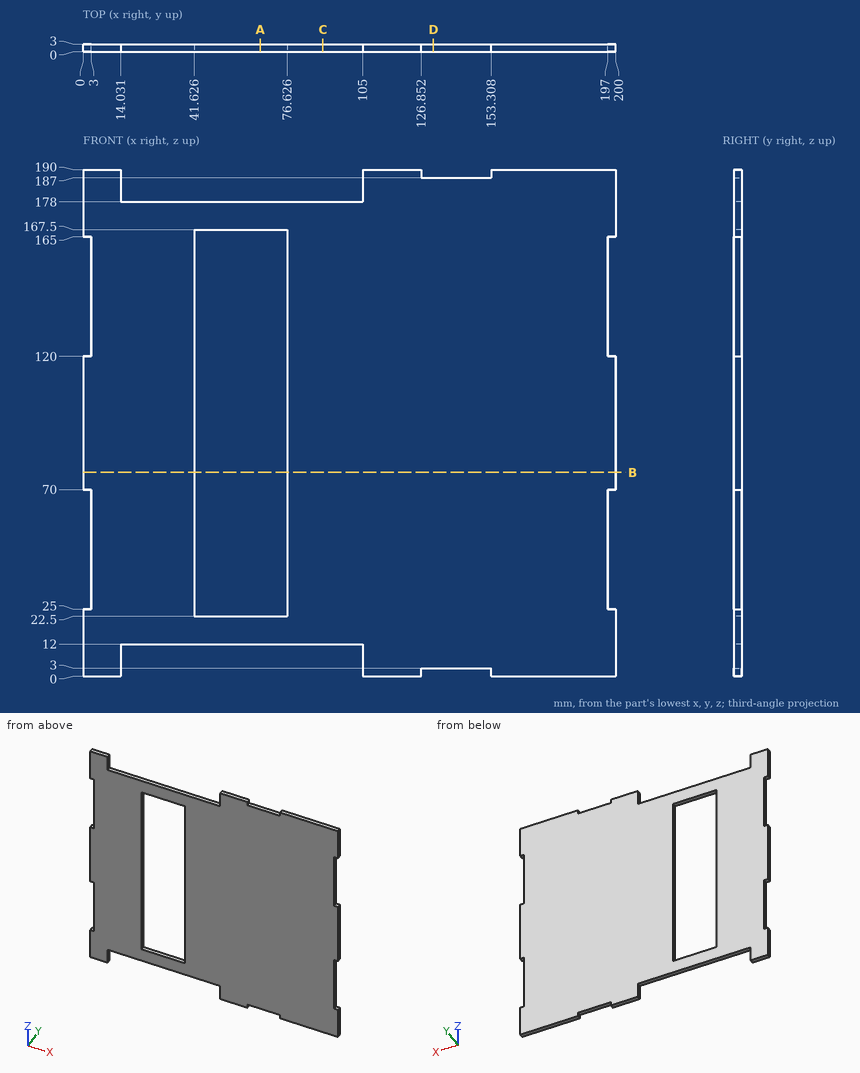
Verification items for this drawing (mm, ordinates from the low corner). Give positions to 0.01 mm unless a question says otherwise; leave off trailing zeros. Write each loop counter-clockwise with the first axis right and the second up, starting at its lowest first coordinate (ties: lowest second). Pieces come first, ordered by that corner, then holes. Notation, with made-up numbers: (40.25, -26) -> (90.25, -26) arc R14 cw to (90.25, -19) -> close; hole circle Ø2 at (26.25, 84.5). An arc over 180 degrees is marked (long way). Use one line per item in the form item = value.
Item 1: Depth check by flat-ended pin: pin 1 Ø1 at (x, y) = (26.5, 2.5) entering from -Z; pin 2 Ø1.5 at (x, y) = (135, 2) entering from +Z; pin 3 Ø1 at (x, y) = (150, 2.5) entering from -Z. Enter the tip coordinate at first touch or a pass-through.
Results list:
pin_1 = 12
pin_2 = 187
pin_3 = 3
Item 2: Sectioned sample at D-D on x = 131.5. Enter the section's corners in (y, z).
Results list:
outline = (0, 3) -> (3, 3) -> (3, 187) -> (0, 187) -> close
Item 3: Sectioned sample at A-A on x = 66.5. Enter the section's corners in (y, z).
Results list:
outline = (0, 12) -> (3, 12) -> (3, 22.5) -> (0, 22.5) -> close; (0, 167.5) -> (3, 167.5) -> (3, 178) -> (0, 178) -> close
Item 4: Sectioned sample at C-C on x = 90. Enter the section's corners in (y, z), plus the area to 3 significant figures.
Results list:
outline = (0, 12) -> (3, 12) -> (3, 178) -> (0, 178) -> close
area = 498 mm2
Item 5: Sectioned sample at B-B on z = 76.5. Enter the section's corners in (x, y), plus the area to 3 significant figures.
Results list:
outline = (0, 0) -> (41.63, 0) -> (41.63, 3) -> (0, 3) -> close; (76.63, 0) -> (200, 0) -> (200, 3) -> (76.63, 3) -> close
area = 495 mm2
Item 6: Scan lines: line 1 (Z direction, x = 60, y = 0.45); line 2 (X direction, y = 0.95, z = 152); line 3 (Z direction, x = 144, y = 0.6). Record each from-to range of solid material in increasing order.
Results list:
line_1 = 12 to 22.5, 167.5 to 178
line_2 = 3 to 41.63, 76.63 to 197
line_3 = 3 to 187
